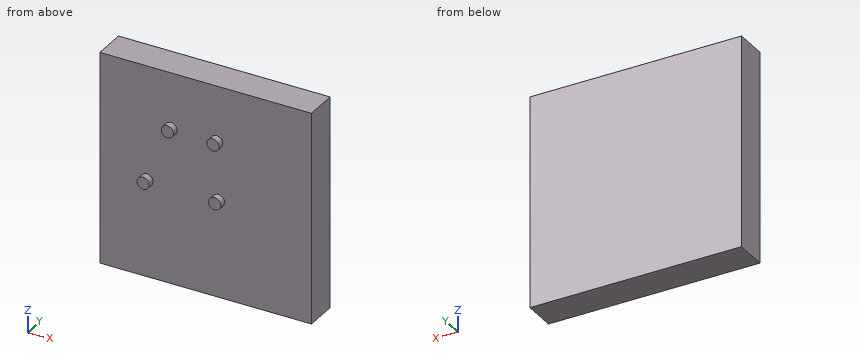
from build123d import *

# Parameters (mm, degrees)
F0_W     = 165.1
F0_H     = 165.1
F1_DEPTH = 25.4
F2_R     = 4.7625
F3_DEPTH = 5.08


with BuildPart() as f1:
    # F0 (on Front) → F1 (new body)
    with BuildSketch(Plane.XZ):
        Rectangle(F0_W, F0_H)
    extrude(amount=F1_DEPTH)

    # F2 (on face) → F3 (join)
    with BuildSketch(Plane.XZ.offset(25.4)):
        with Locations((-26.999259, 38.942747)):
            Circle(F2_R)
        with Locations((8.560741, 38.942747)):
            Circle(F2_R)
        with Locations((-45.89247, -6.777253)):
            Circle(F2_R)
        with Locations((9.98753, -6.777253)):
            Circle(F2_R)
    extrude(amount=F3_DEPTH)


solid = f1.part
The listing builds one solid part. Answer for the finished solid, in the listing's coordinates (mm). Give positions to 0.01 mm unless a question says otherwise; leave off trailing zeros. Order: outer loops, then holes, each group sorted by start corner. A loop starts at its lowest first (then second) coordinate and runs counter-clockwise, first axis right, second up. Notation, with made-up numbers: (-6.75, 84) - (45.25, 84) arc R31 cw to (45.25, 108) - close; hole circle Ø4 at (41, -13.75). An arc over 180 degrees is marked (long way). Answer as CSV lines item,"result".
Q1. A straight line is drawn through the part: L1, parallel to Y at x = -27, z = -65. Find the intervals that lie inside material, in ascending order.
Answer key:
L1,"y = -25.4 to 0"
Q2. A cutting plane is placed at B-B, the plane z = -34. Determine the outline of the cut face in (x, y).
Answer key:
outline,"(-82.55, -25.4) - (82.55, -25.4) - (82.55, 0) - (-82.55, 0) - close"
Q3. A cutting plane is placed at C-C, the plane x = 39.5. Determine the outline of the cut face in (y, z), and give its area (3 significant figures).
Answer key:
outline,"(-25.4, -82.55) - (0, -82.55) - (0, 82.55) - (-25.4, 82.55) - close"
area,"4,190 mm^2"
Q4. A cutting plane is placed at A-A, the plane x = -27. Determine the outline of the cut face in (y, z), and give its area (3 significant figures).
Answer key:
outline,"(-30.48, 34.18) - (-25.4, 34.18) - (-25.4, -82.55) - (0, -82.55) - (0, 82.55) - (-25.4, 82.55) - (-25.4, 43.71) - (-30.48, 43.71) - close"
area,"4,240 mm^2"
Q5. Each of these flat-tipped pins is pushed along its axis until it touches: pin 1 Ø1 at (x, y) = (4, -26) entering from -Z; pin 2 Ø8 at (x, z) = (9.5, 57.5) entering from -Y. Where does it stop, or does it pass through?
Answer key:
pin 1,"stops at z = 36.45"
pin 2,"stops at y = -25.4"
